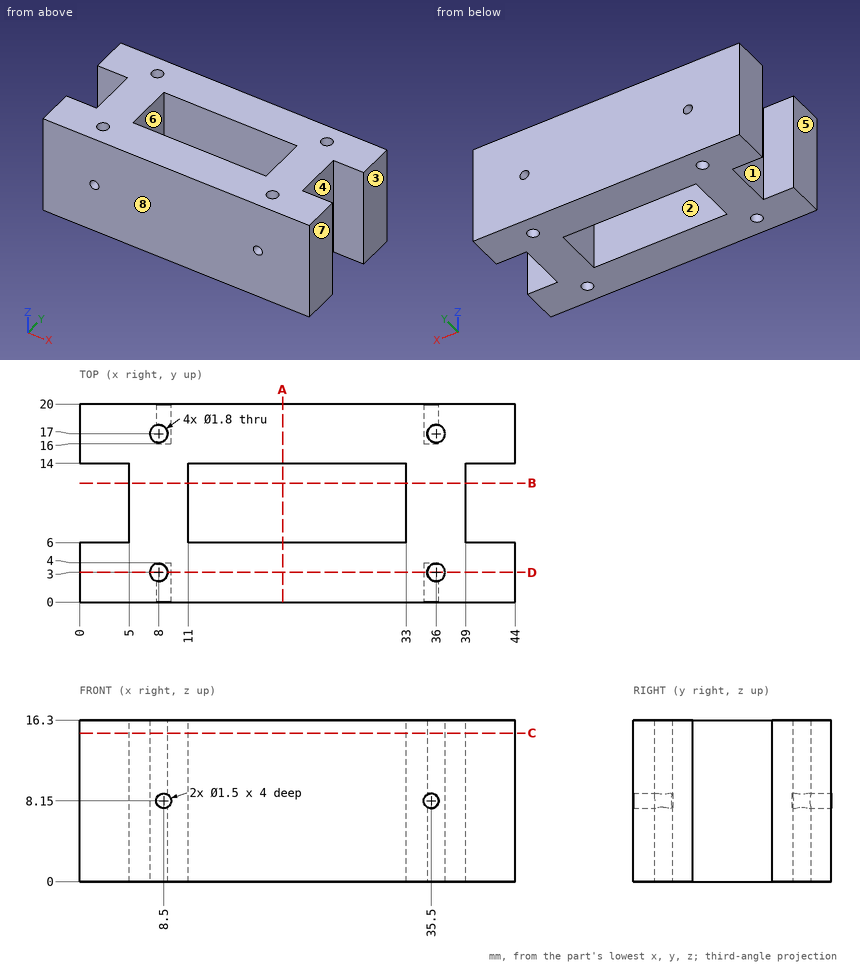
Geometry check sheet. Reference: drawing and pictorial views, mm from the part's lowest x, y, z. A direction names the side the tool comes from. Round coordinates to 2 decimals unless told otherwise and drop trailing zeros. Write each loop counter-clockwise with the first axis right and the second up, starting at its lowest first coordinate (ties: lowest second). Pieces come first, ordered by that corner, then holes.
(1) Access from +Z, -Z, +X, -X, +Y, -Y to the whole of each face (thin tool, end or side, straight path). Record for the marked faces 1, 2, 3, 4 and 5.
Returned:
face 1: +Z, -Z, -X
face 2: +Z, -Z
face 3: +Z, -Z, +X, +Y, -Y
face 4: +Z, -Z, +X
face 5: +Z, -Z, -X, +Y, -Y
(2) Material ranges on line 1 (Y direction, x = 8, z = 3.5); line 2 (Y direction, x = 18, z = 13.25); line 3 (X direction, y = 7, z = 12.25), recorded low to high.
Returned:
line 1: y = 0 to 2.1, 3.9 to 16.1, 17.9 to 20
line 2: y = 0 to 6, 14 to 20
line 3: x = 5 to 11, 33 to 39
(3) Mould release check, pull along Y, two halves, no side actions. Record for the marked faces 6, 7 and 8: pulls with the +Y half, pulls with the -Y half, needs draft (parallel to the pull), parting line crosses it, or undercut.
Returned:
face 6: undercut
face 7: needs draft
face 8: pulls with the -Y half
(4) Section check D-D (y = 3). Enter the section's corners in (x, z), plus the area to 3 significant figures.
Returned:
outline: (0, 0) - (7.1, 0) - (7.1, 16.3) - (0, 16.3) - close; (8.9, 0) - (35.1, 0) - (35.1, 7.52) arc R0.75 cw to (35.1, 8.78) - (35.1, 16.3) - (8.9, 16.3) - (8.9, 8.78) arc R0.75 cw to (8.9, 7.52) - close; (36.9, 0) - (44, 0) - (44, 16.3) - (36.9, 16.3) - close
area: 658 mm2
(5) Section check A-A (x = 20.5). Enter the section's corners in (y, z).
Returned:
outline: (0, 0) - (6, 0) - (6, 16.3) - (0, 16.3) - close; (14, 0) - (20, 0) - (20, 16.3) - (14, 16.3) - close
(6) Depth check by flat-ended pin: pin 1 Ø1.5 at (y, z) = (9, 6.5) entering from +X; pin 2 Ø1.4 at (x, z) = (35.5, 8.15) entering from +Y; pin 3 Ø1.6 at (x, y) = (36, 17) entering from +Z. Enter the tip coordinate at first touch or a pass-through.
Returned:
pin 1: stops at x = 39
pin 2: stops at y = 16
pin 3: passes through
(7) Section check B-B (y = 12). Enter the section's corners in (x, z).
Returned:
outline: (5, 0) - (11, 0) - (11, 16.3) - (5, 16.3) - close; (33, 0) - (39, 0) - (39, 16.3) - (33, 16.3) - close
(8) Section check C-C (z = 15). Enter the section's corners in (x, y).
Returned:
outline: (0, 0) - (44, 0) - (44, 6) - (39, 6) - (39, 14) - (44, 14) - (44, 20) - (0, 20) - (0, 14) - (5, 14) - (5, 6) - (0, 6) - close; hole circle Ø1.8 at (8, 3); hole circle Ø1.8 at (8, 17); hole (11, 6) - (33, 6) - (33, 14) - (11, 14) - close; hole circle Ø1.8 at (36, 3); hole circle Ø1.8 at (36, 17)
